Verification items for the finished model (mm, model axes). A direction names the side the tool comes from. Round coordinates to 2 decimals unless told otherwise and drop trailing zeros. Write each loop counter-clockwise with the first axis right and the second up, starting at its lowest first coordinate (ties: lowest second). Pieces come first, ordered by that corner, then holes. Notation, with made-up numbers: M 75.5,8.5 L 103.5,8.5 A16 cw 103.5,34.5 Z; hole C -6,10.25 d4. An arc over 180 degrees is marked long. Write each question's results on one line, items separated by ' | '.
from build123d import *

# Parameters (mm, degrees)
SKETCH1_W            = 60
SKETCH1_H            = 70
BOSS_EXTRUDE1_DEPTH  = 60
SKETCH2_W            = 60
SKETCH2_H            = 25
CUT_EXTRUDE1_DEPTH   = 9
M5_CLEARANCE_HOLE1_D = 5.5
SKETCH12_R           = 6.75
CUT_EXTRUDE2_DEPTH   = 25


with BuildPart() as part:
    # Sketch1 → Boss-Extrude1 (new body)
    with BuildSketch(Plane.XY):
        with Locations((-30, 35)):
            Rectangle(SKETCH1_W, SKETCH1_H)
    extrude(amount=BOSS_EXTRUDE1_DEPTH)

    # Sketch2 → Cut-Extrude1 (cut)
    with BuildSketch(Plane(origin=(0, 0, 0), x_dir=(0, 0, -1), z_dir=(1, 0, 0))):
        with Locations((-30, 12.5)):
            Rectangle(SKETCH2_W, SKETCH2_H)
    extrude(amount=-CUT_EXTRUDE1_DEPTH, mode=Mode.SUBTRACT)

    # M5 Clearance Hole1 (through all)
    with Locations(Plane(origin=(-9, 10, 35), x_dir=(0, 0, 1), z_dir=(1, 0, 0))):
        with Locations((0, 0), (-16, 0)):
            Hole(M5_CLEARANCE_HOLE1_D / 2)

    # Sketch12 → Cut-Extrude2 (cut)
    with BuildSketch(Plane.ZY.offset(60)):
        with Locations((19, 10)):
            Circle(SKETCH12_R)
        with Locations((35, 10)):
            Circle(SKETCH12_R)
    extrude(amount=-CUT_EXTRUDE2_DEPTH, mode=Mode.SUBTRACT)


solid = part.part
1) Sectioned sample at C-C, the plane x = -53. Record the cut outline in (y, z).
Calculated:
outline: M 0,0 L 70,0 L 70,60 L 0,60 Z; hole C 10,19 d13.5; hole C 10,35 d13.5
2) Draft check along Y on faces 4 (the cylindrical face through (-47.675, 10.297, 28.257)), 5 (the flat face through (-60, 35, 30)), 6 (the flat face through (-35, 7, 19)), 7 (the flat face through (-35, 0, 30)). Enter one of: pulls with the +Y half, pulls with the -Y half, needs draft (parallel to the pull), parting line crosses it, or undercut.
Calculated:
face 4: undercut | face 5: needs draft | face 6: undercut | face 7: pulls with the -Y half
3) Sectioned sample at D-D, the plane z = 55. Record the cut outline in (x, y), and give its area (4 significant figures).
Calculated:
outline: M -60,0 L -9,0 L -9,25 L 0,25 L 0,70 L -60,70 Z | area: 3,975 mm²
4) Depth check by flat-ended pin: P1, Ø21.5, axis at y = 10, z = 19, coming from the +X side; P2, Ø2.5, axis at x = -4, z = 18.5, coming from the -Y side; P3, Ø4.5, axis at y = 10, z = 35, coming from the -X side; P4, Ø4, axis at y = 7, z = 19, coming from the -X side. Enter the tip coordinate at first touch or a pass-through.
Calculated:
P1: stops at x = -9 | P2: stops at y = 25 | P3: passes through | P4: stops at x = -35
5) Material ranges on line 1 (Z direction, x = -18, y = 10); line 2 (Y direction, x = -45, z = 19); line 3 (Z direction, x = -33, y = 11), recorded low to high. Write a range as [from, to].
Calculated:
line 1: z = [0, 16.25], [21.75, 32.25], [37.75, 60] | line 2: y = [0, 3.25], [16.75, 70] | line 3: z = [0, 16.44], [21.56, 32.44], [37.56, 60]
6) Sectioned sample at A-A, the plane z = 35. Record the cut outline in (x, y), and give its area (3 significant figures).
Calculated:
outline: M -60,0 L -9,0 L -9,7.25 L -35,7.25 L -35,3.25 L -60,3.25 Z; M -60,16.75 L -35,16.75 L -35,12.75 L -9,12.75 L -9,25 L 0,25 L 0,70 L -60,70 Z | area: 3,490 mm²
7) Access from +Z, -Z, +X, -X, +Y, -Y to the whole of each face (thin tool, end or side, straight path). Record for faces 1 (the cylindrical face through (-47.675, 12.028, 25.438)), 2 (the cylindrical face through (-22.182, 9.879, 21.747)), 3 (the flat face through (-9, 13, 30)).
Calculated:
face 1: -X | face 2: +X, -X | face 3: +Z, -Z, +X, -Y
8) Sectioned sample at B-B, the plane y = 10. Record the cut outline in (x, z), and give its area (3 significant figures).
Calculated:
outline: M -60,0 L -9,0 L -9,16.25 L -35,16.25 L -35,12.25 L -60,12.25 Z; M -60,25.75 L -35,25.75 L -35,21.75 L -9,21.75 L -9,32.25 L -35,32.25 L -35,28.25 L -60,28.25 Z; M -60,41.75 L -35,41.75 L -35,37.75 L -9,37.75 L -9,60 L -60,60 Z | area: 2,100 mm²
